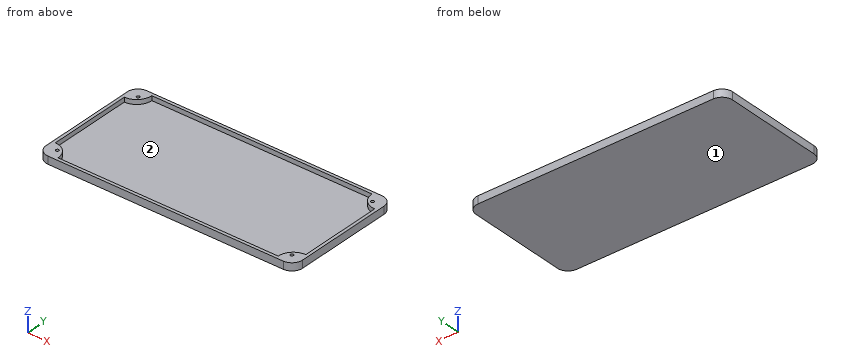
```python
from build123d import *

# Parameters (mm, degrees)
PAD_DEPTH               = 3
THICKNESS_T             = 2
SKETCH001_R             = 1
PAD001_DEPTH            = 3
SKETCH001_MIRRORED_2_R  = 1
PAD001_MIRRORED_2_DEPTH = 3


with BuildPart() as part:
    # Sketch → Pad (new body)
    with BuildSketch(Plane.XY):
        with BuildLine():
            ThreePointArc((-77.75, 37.75), (-81.285534, 36.285534), (-82.75, 32.75))
            Line((-82.75, -32.75), (-82.75, 32.75))
            ThreePointArc((-82.75, -32.75), (-81.285534, -36.285534), (-77.75, -37.75))
            Line((77.75, -37.75), (-77.75, -37.75))
            ThreePointArc((77.75, -37.75), (81.285534, -36.285534), (82.75, -32.75))
            Line((82.75, 32.75), (82.75, -32.75))
            ThreePointArc((82.75, 32.75), (81.285534, 36.285534), (77.75, 37.75))
            Line((-77.75, 37.75), (77.75, 37.75))
        make_face()
    extrude(amount=PAD_DEPTH)

    # Thickness
    thickness_openings = [part.faces().sort_by_distance(p)[0] for p in [
        (0, 0, 3),
    ]]
    offset(amount=THICKNESS_T, openings=thickness_openings, kind=Kind.INTERSECTION)

    # Sketch001 (on Face9 of Thickness) → Pad001 (join)
    with BuildSketch(Plane.XY):
        with BuildLine():
            Line((-82.75, 32.75), (-82.75, 27.75))
            ThreePointArc((-82.75, 27.75), (-75.678932, 30.678932), (-72.75, 37.75))
            Line((-77.75, 37.75), (-72.75, 37.75))
            ThreePointArc((-77.75, 37.75), (-81.285534, 36.285534), (-82.75, 32.75))
        make_face()
        with Locations((-77.5, 32.5)):
            Circle(SKETCH001_R, mode=Mode.SUBTRACT)
    pad001 = extrude(amount=PAD001_DEPTH)

    # Sketch001 Mirrored 2 → Pad001 Mirrored 2 (add)
    with BuildSketch(Plane(origin=(0, 0, 0), x_dir=(-1, 0, 0), z_dir=(0, 0, -1))):
        with BuildLine():
            Line((-82.75, 32.75), (-82.75, 27.75))
            ThreePointArc((-82.75, 27.75), (-75.678932, 30.678932), (-72.75, 37.75))
            Line((-77.75, 37.75), (-72.75, 37.75))
            ThreePointArc((-77.75, 37.75), (-81.285534, 36.285534), (-82.75, 32.75))
        make_face()
        with Locations((-77.5, 32.5)):
            Circle(SKETCH001_MIRRORED_2_R, mode=Mode.SUBTRACT)
    pad001_mirrored_2 = extrude(amount=-PAD001_MIRRORED_2_DEPTH)

    # Mirrored001: Pad001, Pad001 Mirrored 2 across Sketch001 H_Axis
    add(pad001.mirror(Plane.ZX))
    add(pad001_mirrored_2.mirror(Plane.ZX))


solid = part.part
```
The listing builds one solid part. Answer for the finished solid, in the listing's coordinates (mm). Face numbers are marked on the shaded views. Coordinates: 2 decimals unless noted, no trailing zeros. Write each loop counter-clockwise with the first axis right and the second up, starting at its lowest first coordinate (ties: lowest second). Pieces come first, ordered by that corner, then holes.
Q1. Given P1, Ø12, axis at x = 6.5, y = 12.5, coming from the +Z side, flat-ended and moving along its own axis, determine where the tip first touches the part or whether it passes through.
Returned:
P1: stops at z = 0
Q2. Section B-B, the plane y = 18.5 is taken. Write down the section's boundary in (x, z).
Returned:
outline: (-84.75, -2) - (84.75, -2) - (84.75, 3) - (82.75, 3) - (82.75, 0) - (-82.75, 0) - (-82.75, 3) - (-84.75, 3) - close
Q3. Section C-C, the plane x = -13.5 is taken. Write down the section's boundary in (y, z), then the cut area to 3 significant figures.
Returned:
outline: (-39.75, -2) - (39.75, -2) - (39.75, 3) - (37.75, 3) - (37.75, 0) - (-37.75, 0) - (-37.75, 3) - (-39.75, 3) - close
area: 171 mm2
Q4. Section A-A, the plane z = 2.1 is taken. Write down the section's boundary in (x, y).
Returned:
outline: (-84.75, -32.75) arc R7 ccw to (-77.75, -39.75) - (77.75, -39.75) arc R7 ccw to (84.75, -32.75) - (84.75, 32.75) arc R7 ccw to (77.75, 39.75) - (-77.75, 39.75) arc R7 ccw to (-84.75, 32.75) - close; hole (-82.75, -27.75) arc R10 cw to (-72.75, -37.75) - (72.75, -37.75) arc R10 cw to (82.75, -27.75) - (82.75, 27.75) arc R10 cw to (72.75, 37.75) - (-72.75, 37.75) arc R10 cw to (-82.75, 27.75) - close; hole circle Ø2 at (-77.5, -32.5); hole circle Ø2 at (-77.5, 32.5); hole circle Ø2 at (77.5, -32.5); hole circle Ø2 at (77.5, 32.5)
Q5. Find the intervals of material crossed by line 1 along Y through (x, z) = (-77.5, 1.9); line 2 along Y through (x, z) = (-63, 2.3); line 3 along X through (y, z) = (-18, 1.75), in increasing order.
Returned:
line 1: y = -39.75 to -33.5, -31.5 to -29.24, 29.24 to 31.5, 33.5 to 39.75
line 2: y = -39.75 to -37.75, 37.75 to 39.75
line 3: x = -84.75 to -82.75, 82.75 to 84.75
Q6. The mould has two halves that part along X. Classify the marked faces 1 and 2: released by +X, released by -X, zero draft, split by the parting line, or undercut.
Returned:
face 1: zero draft
face 2: undercut
